Here's the drawing with two shaded views (mm, measured from the low corner). I have some questions. A direction names the side the tool comes from. Give positions to 0.01 mm unless a question says otherwise; leave off trailing zeros. Order: outer loops, then holes, each group sorted by start corner. A loop starts at its lowest first (then second) coordinate and runs counter-clockwise, first axis right, second up. Notation, with made-up numbers: M 88.5,-16 L 100.5,-16 A23 ccw 100.5,13 Z; hole C 51.5,13 d4. An arc over 180 degrees is marked long. Write each question's results on one line, items separated by ' | '.
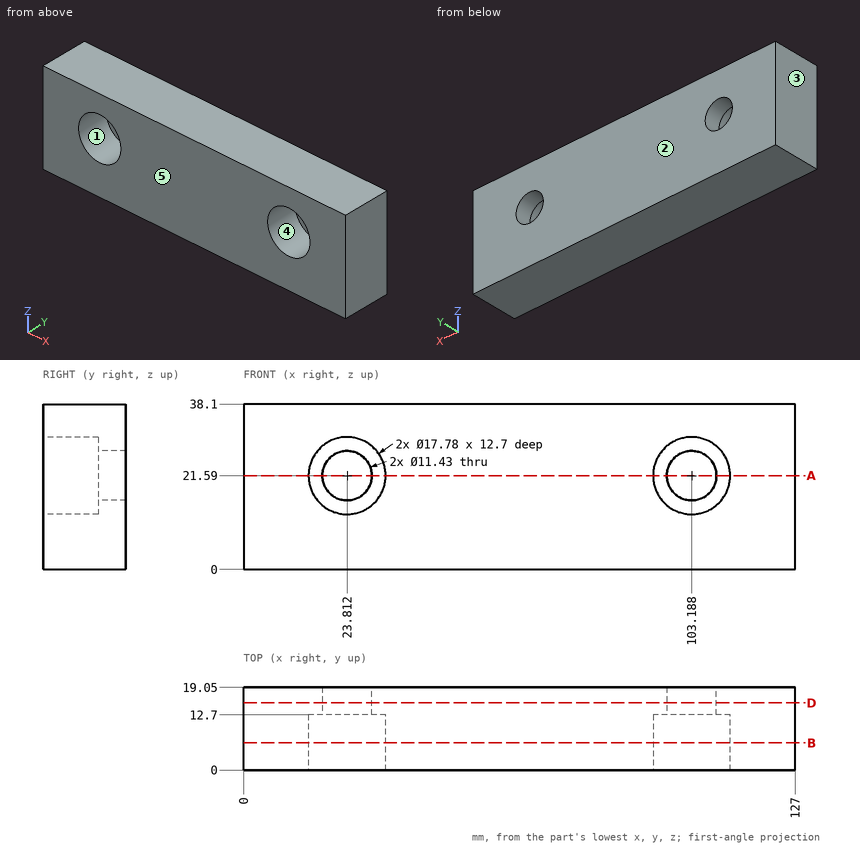
(1) For the marked faces 1 and 2, which set-ups out of +Z, -Z, +X, -X, +Y, -Y let a thin tool reach every point of the face, with its end or its side?
Data:
face 1: -Y | face 2: +Z, -Z, +X, -X, +Y
(2) Will these pins go through, and if not, where does the flat tip stop? P1, Ø1.5, axis at x = 21, y = 14, coming from the -Z side; P2, Ø10.5, axis at x = 23.81, z = 21.59, coming from the -Y side.
Data:
P1: stops at z = 0 | P2: passes through
(3) We'd pull the mould along X, two halves only. Please class the marked faces 3, 4 and 5: +X half, -X half, draft (parallel to the pull), parting line (faces both ways), or undercut.
Data:
face 3: -X half | face 4: undercut | face 5: draft
(4) Imagine slicing it at A-A, the plane z = 21.59. Write out the boundary of the cut face in (x, y), plus the area to 3 significant figures.
Data:
outline: M 0,0 L 14.92,0 L 14.92,12.7 L 18.1,12.7 L 18.1,19.05 L 0,19.05 Z; M 29.53,12.7 L 32.7,12.7 L 32.7,0 L 94.3,0 L 94.3,12.7 L 97.47,12.7 L 97.47,19.05 L 29.53,19.05 Z; M 108.9,12.7 L 112.08,12.7 L 112.08,0 L 127,0 L 127,19.05 L 108.9,19.05 Z | area: 1,820 mm2
(5) Imagine slicing it at B-B, the plane y = 6.25. Write out the boundary of the cut face in (x, z).
Data:
outline: M 0,0 L 127,0 L 127,38.1 L 0,38.1 Z; hole C 23.81,21.59 d17.78; hole C 103.19,21.59 d17.78
(6) Imagine slicing it at D-D, the plane y = 15.5. Write out the boundary of the cut face in (x, z) (1 decimal), plus the area to 3 significant figures.
Data:
outline: M 0,0 L 127,0 L 127,38.1 L 0,38.1 Z; hole C 23.8,21.6 d11.4; hole C 103.2,21.6 d11.4 | area: 4,630 mm2
(7) I need wall thicknesses on L1, parallel to X at y = 16.75, z = 21.59; L2, parallel to X at y = 2.5, z = 20 (1 decimal); L3, parallel to Y at x = 18, z = 23.5. Which ranges of each line are inside material? Lowest first, please. Write a range as from..to.
Data:
L1: x = 0..18.1, 29.53..97.47, 108.9..127 | L2: x = 0..15.1, 32.6..94.4, 111.9..127 | L3: y = 12.7..19.05
